```python
from build123d import *

# Parameters (mm, degrees)
SKETCH2_R               = 2.54
CUT_EXTRUDE2_DEPTH      = 5.8260001
CUT_EXTRUDE2_DEPTH_BACK = 5.8260001


with BuildPart() as part:
    # Sketch1 → Revolve1 (revolve)
    with BuildSketch(Plane(origin=(0, 0, 0), x_dir=(0, 0, -1), z_dir=(1, 0, 0))):
        with BuildLine():
            Line((2.54, 0), (11.303, 0))
            Line((11.303, 0), (12.319, 0))
            ThreePointArc((12.319, 0), (12.085657597, 2.470822652), (11.303, 4.826))
            Line((11.303, 4.826), (-11.303, 4.826))
            Line((-11.303, 4.826), (-11.303, 2.794))
            Line((-11.303, 2.794), (-29.845, 2.794))
            Line((-29.845, 2.794), (-29.845, 1.524))
            Line((-29.845, 1.524), (-11.303, 1.524))
            Line((-11.303, 1.524), (-11.303, 0))
            Line((-11.303, 0), (-2.54, 0))
            ThreePointArc((-2.54, 0), (0, 2.54), (2.54, 0))
        make_face()
    revolve(axis=Axis((0, 0, 36.613472311), (0, 0, -1)))

    # Sketch2 → Cut-Extrude2 (cut, two sides)
    with BuildSketch(Plane(origin=(0, 0, 0), x_dir=(0, 0, -1), z_dir=(1, 0, 0))) as cut_extrude2_sk:
        Circle(SKETCH2_R)
    extrude(amount=CUT_EXTRUDE2_DEPTH, mode=Mode.SUBTRACT)
    extrude(cut_extrude2_sk.sketch, amount=-CUT_EXTRUDE2_DEPTH_BACK, mode=Mode.SUBTRACT)


solid = part.part
```
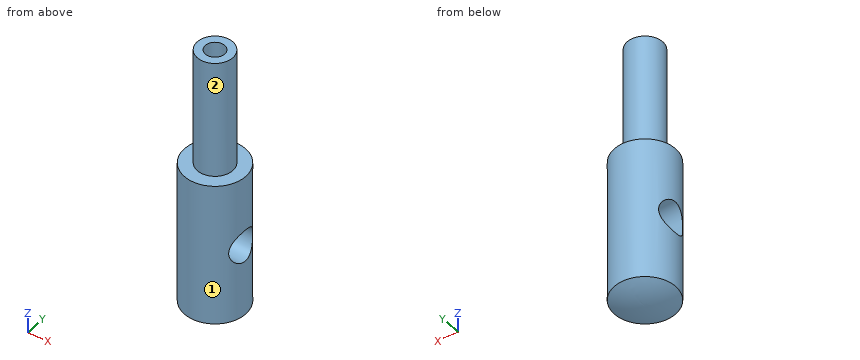
CAD build for the part. Positions are in the model's coordinates, mm. Face numbers are marked on the shaded views. A direction names the side the tool comes from. Give positions to 0.01 mm unless a question says otherwise; leave off trailing zeros. Write each loop counter-clockwise with the first axis right and the second up, starting at its lowest first coordinate (ties: lowest second). Pieces come first, ordered by that corner, then holes. Notation, with made-up numbers: M 30,67.5 L 87,67.5 A34 cw 87,99.5 Z; hole C 18.5,55.5 d11. An arc over 180 degrees is marked long. Return JSON: item names as keys, results as strings. Group by question number.
(1) Flat gauge pins, fed straight in: pin 1 Ø2 at (x, z) = (0.5, 17) entering from +Y; pin 2 Ø3 at (y, z) = (0, 0) entering from -X; pin 3 Ø3 at (y, z) = (-2, -2) entering from +X; pin 4 Ø5 at (x, z) = (-3.5, 6) entering from -Y. Where does each tip first touch, or does it go through?
(2) 3-axis set-ups, long thin cutter, end or side, ignore diameter. For the marked faces 1 and 2: which of +Z, -Z, +X, -X, +Y, -Y reach the whole face in a straight line?
(3) Band-saw the part on B-B (z = 0). Give the cut face in (x, y).
(4) Drill centre lines: L1, parallel to Y at x = -3.75, z = 0; L2, parallel to Z at x = 2.25, y = 2.25; L3, parallel to Z at x = 3, y = -1. Where is each one in solid material? Low to high. Write a range as [from, to].
(5) Band-saw the part on C-C (z = -5). Give the cut face in (x, y).
(6) Band-saw the part on A-A (z = 25.5). Give the cut face in (x, y), and give its area (3 significant figures).
Entries:
{
 "1": {"pin 1": "stops at y = 2.79", "pin 2": "passes through", "pin 3": "stops at x = 4.79", "pin 4": "stops at y = -4.72"},
 "2": {"face 1": "+Z, -Z", "face 2": "+Z"},
 "3": {"outline": "M -4.1,-2.54 A4.83 ccw 4.1,-2.54 Z; M -4.1,2.54 L 4.1,2.54 A4.83 ccw Z"},
 "4": {"L1": "y = [-3.04, -2.54], [2.54, 3.04]", "L2": "z = [-11.91, -1.18], [1.18, 11.3]", "L3": "z = [-11.92, -2.33], [2.33, 11.3]"},
 "5": {"outline": "C 0,0 d9.65"},
 "6": {"outline": "C 0,0 d5.59; hole C 0,0 d3.05", "area": "17.2 mm^2"}
}
